Read the model definition and answer for the solid it produces. Units are mm, in the model's axes. A direction names the side the tool comes from. Coordinates: 2 decimals unless noted, no trailing zeros. Write each loop counter-clockwise with the first axis right and the second up, starting at its lowest first coordinate (ties: lowest second). Pieces come first, ordered by that corner, then holes. Notation, with made-up numbers: (33, 8) - (43, 8) arc R10 cw to (43, 23) - close; hole circle Ø9 at (39.5, -25). An arc over 180 degrees is marked (long way). Return JSON: item names as keys, results as strings.
```python
from build123d import *

# Parameters (mm, degrees)
F1_DEPTH = 5.715


with BuildPart() as f1:
    # F0 (on Top) → F1 (new body)
    with BuildSketch(Plane.XY):
        with BuildLine():
            Line((8.89, 9.652), (0, 9.652))
            Line((0, 9.652), (0, 6.4135))
            ThreePointArc((0, 6.4135), (1.5875, 4.826), (0, 3.2385))
            Line((0, 3.2385), (0, 0))
            Line((0, 0), (8.89, 0))
            Line((8.89, 0), (8.89, 2.413))
            ThreePointArc((8.89, 2.413), (8.021609, 3.617828), (6.604, 3.175))
            Line((6.604, 3.175), (2.794, 3.175))
            Line((2.794, 3.175), (2.794, 6.477))
            Line((2.794, 6.477), (6.604, 6.477))
            ThreePointArc((6.604, 6.477), (8.021609, 6.034172), (8.89, 7.239))
            Line((8.89, 7.239), (8.89, 9.652))
        make_face()
    extrude(amount=F1_DEPTH)


solid = f1.part
```
(1) Straight lines are drawn through the part: line 1 (Y direction, x = 5.25, z = 4.75) (3 decimals); line 2 (X direction, y = 4.75, z = 5.15); line 3 (Y direction, x = 7.25, z = 5.4). For each, find the intervals that lie inside material, in ascending order. Write a range as from..to.
Answer:
{"line 1": "0..3.175, 6.477..9.652", "line 2": "1.59..2.79", "line 3": "0..3.63, 6.02..9.65"}
(2) A cutting plane is placed at C-C (x = 7). Determine the outline of the cut face in (y, z) (3 decimals).
Answer:
{"outline": "(0, 0) - (3.521, 0) - (3.521, 5.715) - (0, 5.715) - close; (6.131, 0) - (9.652, 0) - (9.652, 5.715) - (6.131, 5.715) - close"}
(3) Determine the mould class of faces 3 (the face through (2, 5, 0)), 4 (the face through (8.89, 1, 3)), 5 (the face through (5, 3.175, 3)) for opening direction X: +X half, -X half, draft (parallel to the pull), parting line (faces both ways), or undercut.
Answer:
{"face 3": "draft", "face 4": "+X half", "face 5": "undercut"}
(4) Which of the six approach directions +Z, -Z, +X, -X, +Y, -Y give full straight-line access (tool end or side, diameter ignored) to faces 1 (the face through (2.794, 5, 3)), 2 (the face through (0, 2, 3))?
Answer:
{"face 1": "+Z, -Z", "face 2": "+Z, -Z, -X, +Y, -Y"}
(5) A flat-ended cylindrical pin translates along its axis: P1, Ø1.7, axis at y = 5.5, z = 1.5, coming from the +X side. Find the tip coordinate at first contact, or state that the pin passes through.
Answer:
{"P1": "x = 8.53"}
(6) A cutting plane is placed at B-B (z = 1.15). Determine the outline of the cut face in (x, y) (1 decimal).
Answer:
{"outline": "(0, 0) - (8.9, 0) - (8.9, 2.4) arc R1.3 ccw to (6.6, 3.2) - (2.8, 3.2) - (2.8, 6.5) - (6.6, 6.5) arc R1.3 ccw to (8.9, 7.2) - (8.9, 9.7) - (0, 9.7) - (0, 6.4) arc R1.6 cw to (0, 3.2) - close"}
(7) A cutting plane is placed at D-D (y = 4.5). Determine the outline of the cut face in (x, z) (3 decimals).
Answer:
{"outline": "(1.554, 0) - (2.794, 0) - (2.794, 5.715) - (1.554, 5.715) - close"}
(8) A cutting plane is placed at A-A (x = 3.5). Determine the outline of the cut face in (y, z) (3 decimals), and give its area (3 significant figures).
Answer:
{"outline": "(0, 0) - (3.175, 0) - (3.175, 5.715) - (0, 5.715) - close; (6.477, 0) - (9.652, 0) - (9.652, 5.715) - (6.477, 5.715) - close", "area": "36.3 mm²"}
